Part model, mm, in its own coordinate system. Round coordinates to 2 decimals unless told otherwise and drop trailing zeros. Write each loop counter-clockwise with the first axis right and the second up, starting at its lowest first coordinate (ties: lowest second). Pieces come first, ordered by that corner, then holes.
1) Saw through at A-A on z = 2.15. Write the cut outline in (x, y).
2) Flat gauge pin, fed straight in: pin 1 (5.5 mm diameter, centred on x = 23, y = 5, fed in from +Z). Where does the tip first touch, or does it go through?
3) Drill centre lines: L1, parallel to X at y = 5, z = 1.15; L2, parallel to X at y = 5, z = 1; L3, parallel to Y at x = 23, z = 0.3. Where is each one in solid material? Low to high.
```python
from build123d import *

# Parameters (mm, degrees)
SKETCH1_W                                      = 335.5
SKETCH1_H                                      = 54
BOSS_EXTRUDE1_DEPTH                            = 3
CHAMFER1_SIZE                                  = 3
CSK_FOR_M3_FLAT_HEAD_MACHINE_SCREW1_AT_2_COUNT = 2
CSK_FOR_M3_FLAT_HEAD_MACHINE_SCREW1_AT_2_PITCH = 100
CSK_FOR_M3_FLAT_HEAD_MACHINE_SCREW1_AT_3_COUNT = 2
CSK_FOR_M3_FLAT_HEAD_MACHINE_SCREW1_AT_3_PITCH = 189.5
CSK_FOR_M3_FLAT_HEAD_MACHINE_SCREW1_AT_4_COUNT = 2
CSK_FOR_M3_FLAT_HEAD_MACHINE_SCREW1_AT_4_PITCH = 289.5


with BuildPart() as part:
    # Sketch1 → Boss-Extrude1 (new body)
    with BuildSketch(Plane.XY):
        with Locations((167.75, 27)):
            Rectangle(SKETCH1_W, SKETCH1_H)
    extrude(amount=BOSS_EXTRUDE1_DEPTH)

    # Chamfer1
    chamfer1_edges = [part.edges().sort_by_distance(p)[0] for p in [
        (0, 27, 0),
        (167.75, 54, 0),
        (335.5, 27, 0),
    ]]
    chamfer(chamfer1_edges, length=CHAMFER1_SIZE - 0.0001)  # a hair under: the kernel refuses the full size

    # Sketch3 → CSK for M3 Flat Head Machine Screw1 (revolve, cut)
    with BuildSketch(Plane(origin=(23, 5, 3), x_dir=(0, -1, 0), z_dir=(1, 0, 0))):
        Polygon((0, 0), (0, 3), (1.7, 3), (1.7, 1.45), (3.15, 0), align=None)
    csk_for_m3_flat_head_machine_screw1 = revolve(axis=Axis((23, 5, 9.35), (0, 0, -1)), mode=Mode.SUBTRACT)

    # CSK for M3 Flat Head Machine Screw1 at 2: CSK for M3 Flat Head Machine Screw1 ×2
    with Locations(*[(i * CSK_FOR_M3_FLAT_HEAD_MACHINE_SCREW1_AT_2_PITCH, 0, 0) for i in range(1, CSK_FOR_M3_FLAT_HEAD_MACHINE_SCREW1_AT_2_COUNT)]):
        add(csk_for_m3_flat_head_machine_screw1, mode=Mode.SUBTRACT)

    # CSK for M3 Flat Head Machine Screw1 at 3: CSK for M3 Flat Head Machine Screw1 ×2
    with Locations(*[(i * CSK_FOR_M3_FLAT_HEAD_MACHINE_SCREW1_AT_3_PITCH, 0, 0) for i in range(1, CSK_FOR_M3_FLAT_HEAD_MACHINE_SCREW1_AT_3_COUNT)]):
        add(csk_for_m3_flat_head_machine_screw1, mode=Mode.SUBTRACT)

    # CSK for M3 Flat Head Machine Screw1 at 4: CSK for M3 Flat Head Machine Screw1 ×2
    with Locations(*[(i * CSK_FOR_M3_FLAT_HEAD_MACHINE_SCREW1_AT_4_PITCH, 0, 0) for i in range(1, CSK_FOR_M3_FLAT_HEAD_MACHINE_SCREW1_AT_4_COUNT)]):
        add(csk_for_m3_flat_head_machine_screw1, mode=Mode.SUBTRACT)


solid = part.part
```
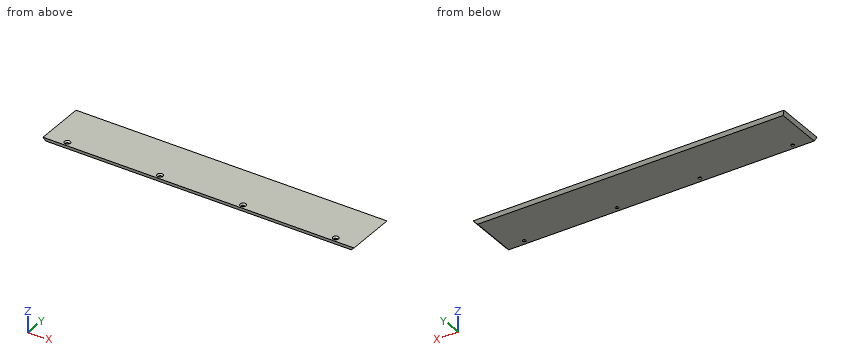
Completed:
1. outline: (0.85, 0) - (334.65, 0) - (334.65, 53.15) - (0.85, 53.15) - close; hole circle Ø4.6 at (23, 5); hole circle Ø4.6 at (123, 5); hole circle Ø4.6 at (212.5, 5); hole circle Ø4.6 at (312.5, 5)
2. pin 1: stops at z = 2.6
3. L1: x = 1.85 to 21.3, 24.7 to 121.3, 124.7 to 210.8, 214.2 to 310.8, 314.2 to 333.65
3. L2: x = 2 to 21.3, 24.7 to 121.3, 124.7 to 210.8, 214.2 to 310.8, 314.2 to 333.5
3. L3: y = 0 to 3.3, 6.7 to 51.3
